The listing builds one solid part. Answer for the finished solid, in the listing's coordinates (mm). A direction names the side the tool comes from. Round coordinates to 2 decimals unless told otherwise and drop trailing zeros. Order: outer loops, then holes, each group sorted by start corner. A loop starts at its lowest first (then second) coordinate and runs counter-clockwise, first axis right, second up. Notation, with made-up numbers: M 33.5,21 L 79.5,21 A18 cw 79.5,51 Z; hole C -8,26.5 d7. An arc over 180 degrees is marked long. Put each result on its own line as item: value. Start each with the question number.
1. The part is cut by section D-D (z = 6.5). Give the vertices of the cut face in (x, y).
2. The part is cut by section C-C (x = 27.5). Give the vertices of the cut face in (y, z), then the cut area to 3 significant figures.
3. The mould has two halves that part along Z. Classify faces 4 (the face through (-2.43, -3.45, 15.33)), 5 (the face through (-0.735, -3.451, -23.426)), 6 (the face through (-5, -7, -13)): +Z half, -Z half, draft (parallel to the pull), parting line (faces both ways), or undercut.
4. Each of these flat-tipped pins is pushed along its axis until it touches: pin 1 Ø4 at (y, z) = (-5, 2.5) entering from -X; pin 2 Ø3 at (y, z) = (-1.5, 15) entering from +X. Where does it stop, or does it pass through?
5. The part is cut by section B-B (x = 0). Give the vertices of the cut face in (y, z), then the cut area to 3 significant figures.
6. Which of the six approach directions +Z, -Z, +X, -X, +Y, -Y give full straight-line access (tool end or side, diameter ignored) to faces 1 (the face through (-14.71, -3.45, 5.39)), 2 (the face through (0, -3.5, 13.2)), 3 (the face through (-5, 0, -13))?
7. The part is cut by section A-A (z = -24.5). Give the vertices of the cut face in (x, y), then the cut area to 3 significant figures.
8. Consider line 1 (Z direction, x = 0, y = -5); line 2 (X direction, y = -3.75, z = -20); line 3 (Z direction, x = 1.5, y = -3.5). Determine where each line is inside the solid, lowest interval first.
from build123d import *

# Parameters (mm, degrees)
F0_R     = 11.2
F1_DEPTH = 7


with BuildPart() as f1:
    # F0 (on Front) → F1 (new body)
    with BuildSketch(Plane.XZ):
        with BuildLine():
            ThreePointArc((1.342519, 13.131551), (9.79697, 8.846433), (13.2, 0))
            ThreePointArc((13.2, 0), (-8.846433, -9.79697), (-1.342519, 13.131551))
            ThreePointArc((-1.342519, 13.131551), (-6.828327, 14.966469), (-11.002825, 18.970789))
            ThreePointArc((-11.002825, 18.970789), (-14.793964, 5.203063), (-22.511932, -6.81176))
            ThreePointArc((-22.511932, -6.81176), (-10.999135, -9.029118), (-5.792273, -19.533867))
            ThreePointArc((-5.792273, -19.533867), (-6.443274, -23.628086), (-8.332066, -27.318466))
            ThreePointArc((-8.332066, -27.318466), (-0.609837, -23.422527), (7.278308, -26.970528))
            ThreePointArc((7.278308, -26.970528), (7.731584, -11.472533), (22.605845, -7.096501))
            ThreePointArc((22.605845, -7.096501), (13.099262, 3.962593), (10.542851, 18.320289))
            ThreePointArc((10.542851, 18.320289), (6.484308, 14.765549), (1.342519, 13.131551))
        make_face()
        with BuildLine():
            ThreePointArc((-1.342519, 13.131551), (0, 13.2), (1.342519, 13.131551))
            ThreePointArc((1.342519, 13.131551), (6.484308, 14.765549), (10.542851, 18.320289))
            ThreePointArc((10.542851, 18.320289), (12.5181, 22.075361), (13.2, 26.263103))
            ThreePointArc((13.2, 26.263103), (-3.808064, 38.901878), (-11.002825, 18.970789))
            ThreePointArc((-11.002825, 18.970789), (-6.828327, 14.966469), (-1.342519, 13.131551))
        make_face()
        with Locations((0, 26.263103)):
            Circle(F0_R, mode=Mode.SUBTRACT)
        with BuildLine():
            ThreePointArc((31.38409, -19.533867), (28.968504, -11.922269), (22.605845, -7.096501))
            ThreePointArc((22.605845, -7.096501), (7.731584, -11.472533), (7.278308, -26.970528))
            ThreePointArc((7.278308, -26.970528), (22.075342, -32.147279), (31.38409, -19.533867))
        make_face()
        with Locations((18.18409, -19.533867)):
            Circle(F0_R, mode=Mode.SUBTRACT)
        with BuildLine():
            ThreePointArc((-5.792273, -19.533867), (-10.999135, -9.029118), (-22.511932, -6.81176))
            ThreePointArc((-22.511932, -6.81176), (-29.849441, -27.041323), (-8.332066, -27.318466))
            ThreePointArc((-8.332066, -27.318466), (-6.443274, -23.628086), (-5.792273, -19.533867))
        make_face()
        with Locations((-18.992273, -19.533867)):
            Circle(F0_R, mode=Mode.SUBTRACT)
    extrude(amount=F1_DEPTH)


solid = f1.part
Resolved:
1. outline: M -14.24,-7 L -11.49,-7 L -11.49,0 L -14.24,0 Z; M 11.49,-7 L 12.05,-7 L 12.05,0 L 11.49,0 Z
2. outline: M -7,-28.89 L 0,-28.89 L 0,-25.75 L -7,-25.75 Z; M -7,-13.32 L 0,-13.32 L 0,-10.18 L -7,-10.18 Z
2. area: 43.9 mm2
3. face 4: undercut
3. face 5: -Z half
3. face 6: draft
4. pin 1: x = -17.22
4. pin 2: x = 10.53
5. outline: M -7,-23.43 L 0,-23.43 L 0,-13.2 L -7,-13.2 Z; M -7,13.2 L 0,13.2 L 0,15.06 L -7,15.06 Z; M -7,37.46 L 0,37.46 L 0,39.46 L -7,39.46 Z
5. area: 98.6 mm2
6. face 1: -X, +Y, -Y
6. face 2: +Y, -Y
6. face 3: +Z, -Z, +X, -X, +Y
7. outline: M -31.22,-7 L -29.03,-7 L -29.03,0 L -31.22,0 Z; M -8.95,-7 L -4.92,-7 L -4.92,0 L -8.95,0 Z; M 4.15,-7 L 8.15,-7 L 8.15,0 L 4.15,0 Z; M 28.22,-7 L 30.41,-7 L 30.41,0 L 28.22,0 Z
7. area: 86.9 mm2
8. line 1: -23.43 to -13.2, 13.2 to 15.06, 37.46 to 39.46
8. line 2: -32.18 to -30.18, -7.8 to 6.99, 29.37 to 31.38
8. line 3: -23.6 to -13.11, 13.11 to 15.16, 37.36 to 39.38
